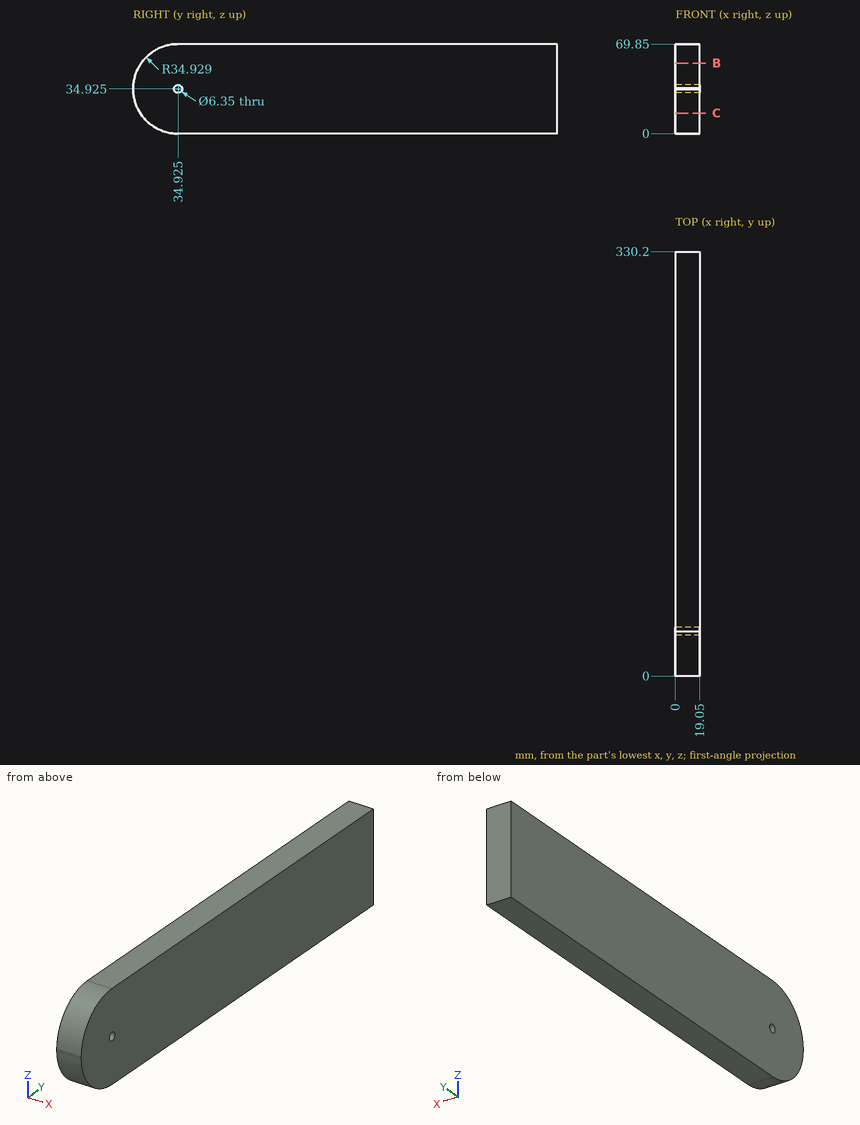
Geometry: see drawing. Coordinates: mm, zero at the bounding-box minimum. Give positions to 0.01 mm unless a question says otherwise; leave off trailing zeros. Order: outer loops, then holes, each group sorted by start corner. A loop starts at its lowest first (then second) coordinate and runs counter-clockwise, first axis right, second up. Notation, with made-up numbers: (32, -37.75) -> (85, -37.75) arc R27 cw to (85, -20.75) -> close; hole circle Ø7 at (16.5, 86.25). An arc over 180 degrees is marked (long way). Write each question's results on one line, items separated by ' | '.
1) Line query: line 1 along Y through (x, z) = (7, 35); line 2 along Y through (x, z) = (9.25, 37.5); line 3 along Y through (x, z) = (7.75, 64.5). Output: solid intervals per line, ascending.
Geometry says:
line 1: y = 0 to 31.75, 38.1 to 330.2 | line 2: y = 0.09 to 33.07, 36.78 to 330.2 | line 3: y = 16.34 to 330.2
2) Cut plane C-C (z = 16). Output: boundary loops of the cut face in (x, y).
Geometry says:
outline: (0, 5.57) -> (19.05, 5.57) -> (19.05, 330.2) -> (0, 330.2) -> close
3) First-contact query: pin 1 Ø1 at (x, z) = (7, 51.5) entering from -Y (1 decimal). Flat tip, straight axial feed; report the tip coordinate or a pass-through.
Geometry says:
pin 1: stops at y = 3.9
4) Cut plane B-B (z = 55). Output: boundary loops of the cut face in (x, y), and give its area (3 significant figures).
Geometry says:
outline: (0, 6.34) -> (19.05, 6.34) -> (19.05, 330.2) -> (0, 330.2) -> close | area: 6,170 mm²
